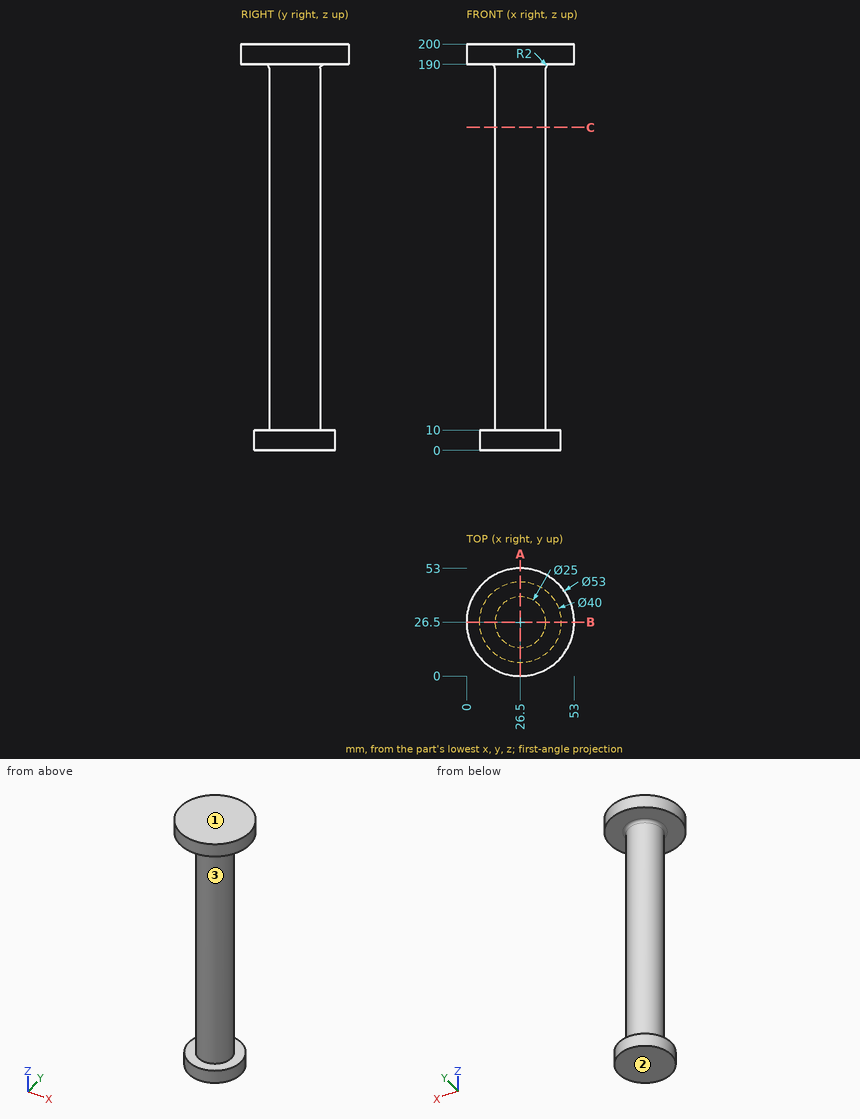
Geometry check sheet. Reference: drawing and pictorial views, mm from the part's lowest x, y, z. Give positions to 0.01 mm unless a question says otherwise; leave off trailing zeros. Write each loop counter-clockwise with the first axis right and the second up, starting at its lowest first coordinate (ties: lowest second). Pieces come first, ordered by that corner, then holes. Notation, with made-up numbers: (88, -39.5) -> (132, -39.5) arc R6 cw to (132, -34.5) -> close; hole circle Ø10 at (6.25, 68.5). An arc over 180 degrees is marked (long way). One line per question, with ' | ' between items.
Item 1: Sectioned sample at A-A, the plane x = 26.5. Record the boundary of the cut face in (y, z), plus the area to 3 significant figures.
Determined:
outline: (0, 190) -> (12, 190) arc R2 cw to (14, 188) -> (14, 10) -> (6.5, 10) -> (6.5, 0) -> (46.5, 0) -> (46.5, 10) -> (39, 10) -> (39, 188) arc R2 cw to (41, 190) -> (53, 190) -> (53, 200) -> (0, 200) -> close | area: 5,430 mm^2
Item 2: Depth check by flat-ended pin: pin 1 (6 mm diameter, centred on x = 29.5, z = 176, fed in from +Y); pin 2 (5 mm diameter, centred on y = 29, z = 77, fed in from -X); pin 3 (4 mm diameter, centred on x = 30, z = 135, fed in from +Y). Enter the tip coordinate at first touch or a pass-through.
Determined:
pin 1: y = 39 | pin 2: x = 14 | pin 3: y = 38.91
Item 3: Scan lines: line 1 along Z through (x, y) = (42, 18); line 2 along Z through (x, y) = (21.5, 2); line 3 along Y through (x, z) = (26, 176). Record each from-to range of solid material in increasing order.
Determined:
line 1: 0 to 10, 190 to 200 | line 2: 190 to 200 | line 3: 14.01 to 38.99
Item 4: Draft check along Z on the marked faces 1, 2 and 3. Enter one of: released by +Z, released by -Z, zero draft, split by the parting line, or undercut.
Determined:
face 1: released by +Z | face 2: released by -Z | face 3: undercut
Item 5: Sectioned sample at C-C, the plane z = 159. Record the boundary of the cut face in (x, y), plus the area to 3 significant figures.
Determined:
outline: circle Ø25 at (26.5, 26.5) | area: 491 mm^2
